Here's how the part is built. I have some questions about the finished solid (model axes, mm). A direction names the side the tool comes from. Give positions to 0.01 mm unless a question says otherwise; leave off trailing zeros. Loops run counter-clockwise (first coordinate to the right, second up) from the corner with the lowest first, then second, coordinate; pieces in that order, holes last. Notation, with made-up numbers: (68.25, -6.5) - (112.25, -6.5) arc R19 ccw to (112.25, 20.5) - close; hole circle Ø9 at (-5.75, 10.25). An arc over 180 degrees is marked (long way). Return JSON: item names as keys, results as strings. Group by question number.
(1) If we section it at D-D (x = -40.5): Please give me the cut outline in (y, z), then the cut area to 3 significant figures.
(2) For P1, Ø4, axis at x = -2, z = 11, coming from the -Y side; P2, Ø8, axis at x = 31.5, y = -26.5, coming from the +Z side; P3, Ø18, axis at x = 26.5, z = 21, coming from the +Y side; P4, Ø13, axis at x = -27, z = 34.5, coming from the +Y side, each with a flat end and sliding along its axis, tell me the tip position at first contact or that it passes through.
(3) If we section it at B-B (x = 36): Please give me the cut outline in (y, z), then the cut area to 3 significant figures.
(4) On a 3-axis mill with a long thin cutter (end or side, diameter ignored), from which of +Z, -Z, +X, -X, +Y, -Y can I reach the whole of each face in a straight line? I mean faces 4 (the cylindrical face through (-1.506, -3.381, 31.219)), 5 (the flat face through (-34, -76.2, 28)), 6 (the flat face through (1, -7.62, 22)), 7 (the flat face through (22.225, -73, 28)), 8 (the cylindrical face through (30.41, -72.981, 53.437)). Say none if no direction works.
(5) If we section it at A-A (y = -50.5): Please give me the cut outline in (x, z) (3 decimals).
(6) If we mould it in two halves opening along Z, with no side actions, what happens to faces 1 (the flat face through (-0.65, 1.85, 21.82)), 2 (the flat face through (30, -69.85, 28)), 3 (the cylindrical face through (30.55, -72.981, 40.683))? For each: released by +Z, released by -Z, zero draft, split by the parting line, or undercut.
(7) I need wall thicknesses on probe 1 along X at (y, z) = (-58, 42) (3 decimals); probe 2 along Y at (x, z) = (14, 26.5); probe 3 along Y at (x, z) = (-32.5, 7). Which ranges of each line are inside material? Lowest first, please. Write a range as [from, to].
(8) If we section it at C-C (z = 34): Please give me the cut outline in (x, y) (3 decimals).
```python
from build123d import *

# Parameters (mm, degrees)
BOSS_EXTRUDE1_DEPTH      = 57.15
CUT_EXTRUDE1_DEPTH       = 102.459011551
BOSS_EXTRUDE2_DEPTH      = 92.71
F_0_257_DIAMETER_HOLE1_D = 6.5278
F_3_0MM_DOWEL_HOLE1_D    = 3.1


with BuildPart() as part:
    # Sketch2 → Boss-Extrude1 (new body)
    with BuildSketch(Plane.XY):
        Polygon((-46.355, 0), (46.355, 0), (46.355, -76.2), (22.225, -76.2), (22.225, -69.85), (38.735, -69.85), (38.735, -7.62), (-38.735, -7.62), (-38.735, -69.85), (-22.225, -69.85), (-22.225, -76.2), (-46.355, -76.2), align=None)
    extrude(amount=BOSS_EXTRUDE1_DEPTH)

    # Sketch3 → Cut-Extrude1 (cut, through all)
    with BuildSketch(Plane(origin=(0, -69.85, 0), x_dir=(1, 0, 0), z_dir=(0, 1, 0))):
        with BuildLine():
            Line((-27.27706, -5.784822778), (-27.27706, -12.134822778))
            ThreePointArc((-27.27706, -12.134822778), (-30.48, -15.337762778), (-33.68294, -12.134822778))
            Line((-33.68294, -12.134822778), (-33.68294, -5.784822778))
            ThreePointArc((-33.68294, -5.784822778), (-30.48, -2.581882778), (-27.27706, -5.784822778))
        make_face()
        with BuildLine():
            Line((-33.68294, -50.234822778), (-33.68294, -43.884822778))
            ThreePointArc((-33.68294, -43.884822778), (-30.48, -40.681882778), (-27.27706, -43.884822778))
            Line((-27.27706, -43.884822778), (-27.27706, -50.234822778))
            ThreePointArc((-27.27706, -50.234822778), (-30.48, -53.437762778), (-33.68294, -50.234822778))
        make_face()
    cut_extrude1 = extrude(amount=-CUT_EXTRUDE1_DEPTH, mode=Mode.SUBTRACT)

    # Mirror1: Cut-Extrude1 across plane
    add(cut_extrude1.mirror(Plane(origin=(0, 0, 0), x_dir=(0, 0, 1), z_dir=(1, 0, 0))), mode=Mode.SUBTRACT)

    # Sketch4 → Boss-Extrude2 (add)
    with BuildSketch(Plane.ZY.offset(46.355)):
        Polygon((57.15, 0), (0, 0), (0, 2.995104586), align=None)
    extrude(amount=-BOSS_EXTRUDE2_DEPTH)

    # F (0.257) Diameter Hole1 (through all)
    with Locations(Plane(origin=(0, 2.986900838, 0.15653684), x_dir=(1, 0, 0), z_dir=(0, 0.9986295347545744, 0.052335956242936806))):
        with Locations((0, -28.457463124)):
            Hole(F_0_257_DIAMETER_HOLE1_D / 2)

    # Ø3.0mm Dowel Hole1 (through all)
    with Locations(Plane(origin=(0, 2.986900838, 0.15653684), x_dir=(1, 0, 0), z_dir=(0, 0.9986295347545744, 0.052335956242936806))):
        with Locations((-18, -28.457463124), (18, -28.457463124)):
            Hole(F_3_0MM_DOWEL_HOLE1_D / 2)


solid = part.part
```
Values:
{
 "1": {"outline": "(-76.2, 0) - (3, 0) - (0, 57.15) - (-76.2, 57.15) - close", "area": "4,440 mm2"},
 "2": {"P1": "y = -7.62", "P2": "through", "P3": "y = 2.37", "P4": "y = 1.53"},
 "3": {"outline": "(-76.2, 0) - (-69.85, 0) - (-69.85, 57.15) - (-76.2, 57.15) - close; (-7.62, 0) - (3, 0) - (0, 57.15) - (-7.62, 57.15) - close", "area": "884 mm2"},
 "4": {"face 4": "none", "face 5": "+Z, -Z, +X, -X, -Y", "face 6": "+Z, -Z", "face 7": "+Z, -Z, -Y", "face 8": "-Y"},
 "5": {"outline": "(-46.355, 0) - (-38.735, 0) - (-38.735, 57.15) - (-46.355, 57.15) - close; (38.735, 0) - (46.355, 0) - (46.355, 57.15) - (38.735, 57.15) - close"},
 "6": {"face 1": "released by +Z", "face 2": "zero draft", "face 3": "undercut"},
 "7": {"probe 1": "[-46.355, -38.735], [38.735, 46.355]", "probe 2": "[-7.62, 1.61]", "probe 3": "[-7.62, 2.63]"},
 "8": {"outline": "(-46.355, -76.2) - (-22.225, -76.2) - (-22.225, -69.85) - (-38.735, -69.85) - (-38.735, -7.62) - (38.735, -7.62) - (38.735, -69.85) - (22.225, -69.85) - (22.225, -76.2) - (46.355, -76.2) - (46.355, 1.213) - (-46.355, 1.213) - close"}
}
